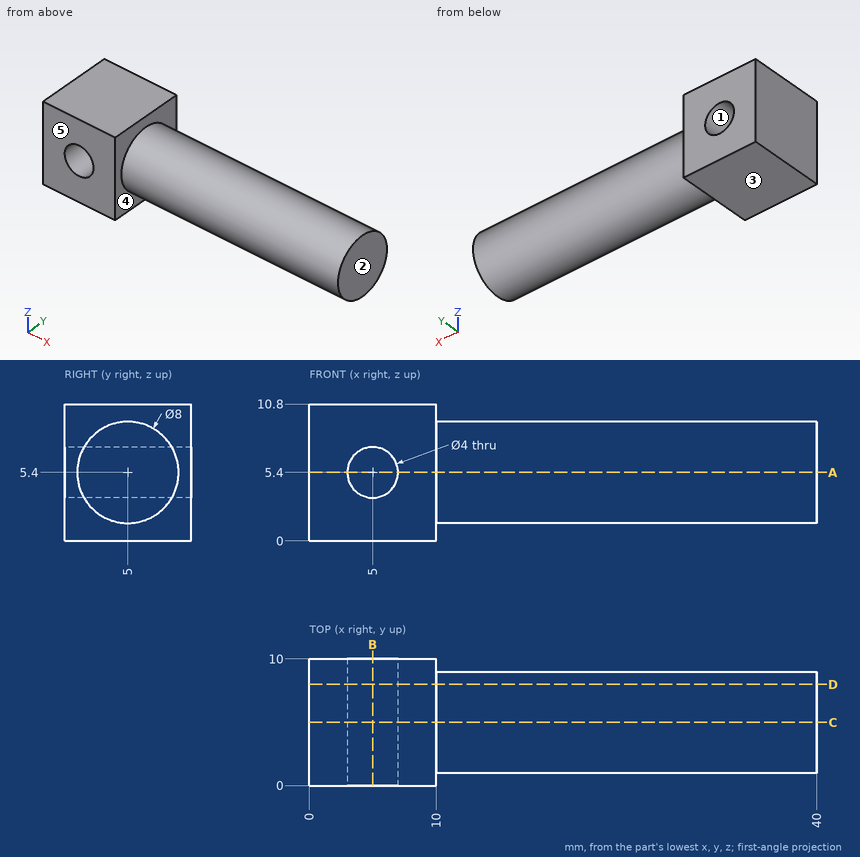
Input: dimensioned drawing with shaded views. Units: mm. Origin: part minimum x, y, z. A direction names the side the tool comes from. Coordinates: 2 decimals unless noted, no trailing zeros. Write each loop counter-clockwise with the first axis right and the second up, starting at its lowest first coordinate (ties: lowest second). Pieces come first, ordered by that corner, then holes. Notation, with made-up numbers: M 41,-1.5 L 47,-1.5 A21 ccw 47,21.5 Z; hole C 82.5,10.5 d1. An arc over 180 degrees is marked long. Answer as CSV lines item,"result". Start each with the question number.
Q1. Cut plane D-D on y = 8. Return the cut outline in (x, z).
Q2. Line query: line 1 (Z direction, x = 5, y = 2.5); line 2 (Y direction, x = 38, z = 5.5); line 3 (X direction, y = 9.5, z = 1.25). Output: solid intervals per line, ascending. Write a range as from..to.
Q3. Cut plane A-A on z = 5.4. Return the cut outline in (x, y).
Q4. Mould query, pull axis Z, two halves, no side actions, for the marked faces 1, 2 and 3. Classes: released by +Z, released by -Z, zero draft, split by the parting line, or undercut.
Q5. Cut plane B-B on x = 5. Return the cut outline in (y, z).
Q6. Pin query (flat end, axial travel): P1, Ø1, axis at x = 26, y = 3.5, coming from the +Z side; P2, Ø1, axis at x = 8.5, y = 9, coming from the -Z side; P3, Ø5, axis at x = 36, y = 9, coming from the -Z side; P4, Ø5, axis at x = 33, z = 6, coming from the +Y side. Return the tip coordinate at first contact, or that it passes through.
Q7. Reachability of the marked faces 4 and 5 from +Z, -Z, +X, -X, +Y, -Y: full face, straight path, thin tool, end or side. Return the list, or none.
Q8. Cut plane C-C on y = 5. Return the cut outline in (x, z).
Findings below:
1,outline,"M 0,0 L 10,0 L 10,2.75 L 40,2.75 L 40,8.05 L 10,8.05 L 10,10.8 L 0,10.8 Z; hole C 5,5.4 d4"
2,line 1,"z = 0..3.4, 7.4..10.8"
2,line 2,"y = 1..9"
2,line 3,"x = 0..10"
3,outline,"M 0,0 L 3,0 L 3,10 L 0,10 Z; M 7,0 L 10,0 L 10,1 L 40,1 L 40,9 L 10,9 L 10,10 L 7,10 Z"
4,face 1,"undercut"
4,face 2,"zero draft"
4,face 3,"released by -Z"
5,outline,"M 0,0 L 10,0 L 10,3.4 L 0,3.4 Z; M 0,7.4 L 10,7.4 L 10,10.8 L 0,10.8 Z"
6,P1,"stops at z = 9.27"
6,P2,"stops at z = 0"
6,P3,"stops at z = 1.69"
6,P4,"stops at y = 9"
7,face 4,"+X"
7,face 5,"+Z, -Z, +X, -X, -Y"
8,outline,"M 0,0 L 10,0 L 10,1.4 L 40,1.4 L 40,9.4 L 10,9.4 L 10,10.8 L 0,10.8 Z; hole C 5,5.4 d4"
